Source: three-view drawing plus pictorial views. Frame: mm from the lowest corner of the part. A direction names the side the tool comes from. Give positions to 0.01 mm unless a question says otherwise; leave off trailing zeros. Write each loop counter-clockwise with the first axis right and the second up, starting at its lowest first coordinate (ties: lowest second). Pieces come first, ordered by that corner, then holes. Notation, with made-up numbers: (-2.75, 62.25) -> (15.25, 62.25) arc R17 ccw to (15.25, 78.25) -> close; hole circle Ø6 at (34, 32.5). An arc over 180 degrees is marked (long way). Write item = value, one per line.
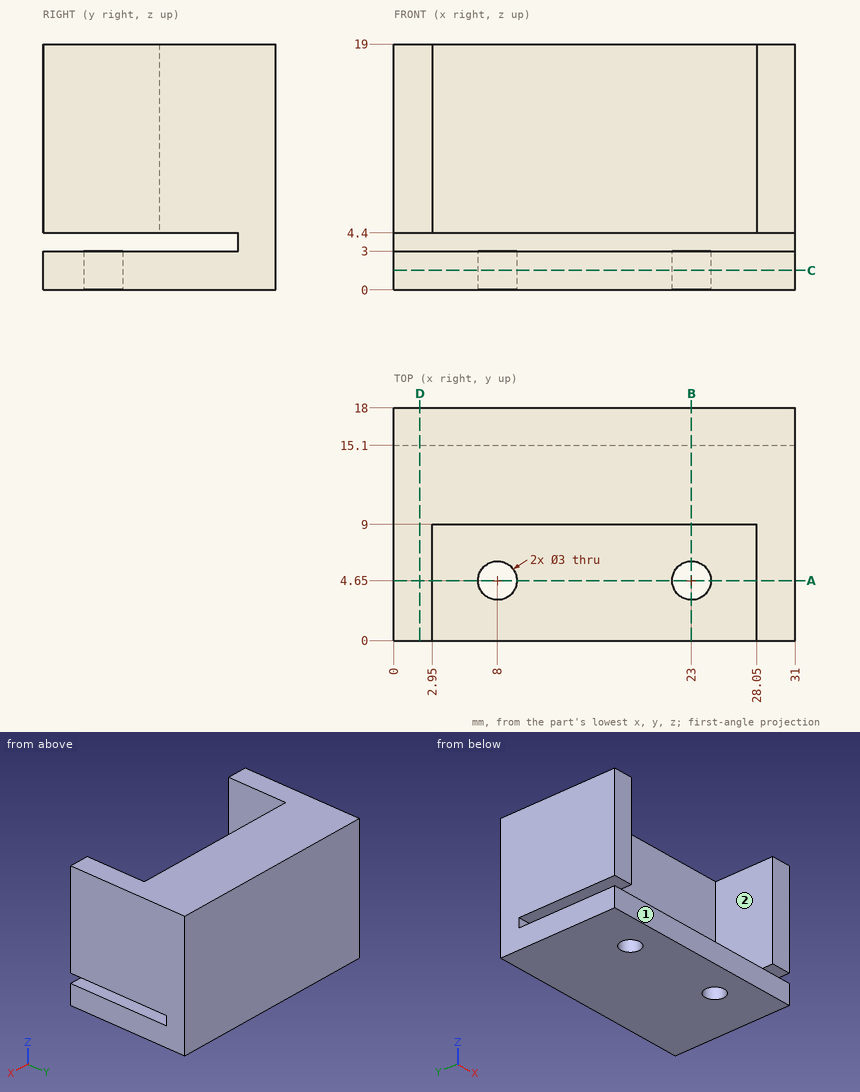
1) Cut plane B-B (x = 23). Return the cut outline in (y, z).
Computed:
outline = (0, 0) -> (3.15, 0) -> (3.15, 3) -> (0, 3) -> close; (6.15, 0) -> (18, 0) -> (18, 19) -> (9, 19) -> (9, 4.4) -> (15.1, 4.4) -> (15.1, 3) -> (6.15, 3) -> close
2) Contact query for flat-ended pins moving along their axis: pin 1 (1.5 mm diameter, centred on x = 20, y = 7, fed in from -Z); pin 2 (2.5 mm diameter, centred on x = 23, y = 4.65, fed in from +Z); pin 3 (2 mm diameter, centred on x = 13, y = 2.5, fed in from +Z); pin 4 (4.5 mm diameter, centred on x = 18.5, z = 12.5, fed in from -Y). Output: stop coordinate, or through.
Computed:
pin_1 = 0
pin_2 = through
pin_3 = 3
pin_4 = 9
3) Access query for the marked faces 1 and 2. Directions: +Z, -Z, +X, -X, +Y, -Y. A direction counts if a zero-diameter tool reaches every point of the face in a straight line with its end or side. Return the directions, or none.
Computed:
face_1 = +Z, -Z, +X, -X, -Y
face_2 = +Z, -Y
4) Cut plane C-C (z = 1.5). Return the cut outline in (x, y).
Computed:
outline = (0, 0) -> (31, 0) -> (31, 18) -> (0, 18) -> close; hole circle Ø3 at (8, 4.65); hole circle Ø3 at (23, 4.65)
5) Cut plane D-D (x = 2). Return the cut outline in (y, z).
Computed:
outline = (0, 0) -> (18, 0) -> (18, 19) -> (0, 19) -> (0, 4.4) -> (15.1, 4.4) -> (15.1, 3) -> (0, 3) -> close
6) Cut plane A-A (y = 4.65). Return the cut outline in (x, z), then the cut area to 3 significant figures.
Computed:
outline = (0, 0) -> (6.5, 0) -> (6.5, 3) -> (0, 3) -> close; (0, 4.4) -> (2.95, 4.4) -> (2.95, 19) -> (0, 19) -> close; (9.5, 0) -> (21.5, 0) -> (21.5, 3) -> (9.5, 3) -> close; (24.5, 0) -> (31, 0) -> (31, 3) -> (24.5, 3) -> close; (28.05, 4.4) -> (31, 4.4) -> (31, 19) -> (28.05, 19) -> close
area = 161 mm²
7) Material intervals for L1, parallel to Z at x = 15, y = 11.5; L2, parallel to X at y = 4.5, z = 6; L3, parallel to Y at x = 23, z = 2.2, sorted ascending.
Computed:
L1 = 0 to 3, 4.4 to 19
L2 = 0 to 2.95, 28.05 to 31
L3 = 0 to 3.15, 6.15 to 18
